Can you work these out from the model? Positions are in its coordinate system, mm. Face numbers are marked on the shaded views. A direction names the side the tool comes from. Give positions to 0.01 mm unless a question says otherwise; leave off trailing zeros. Order: outer loops, then holes, each group sorted by start corner. A loop starts at its lowest first (then second) coordinate and runs counter-clockwise, first axis right, second up. Notation, with made-up numbers: (-30.5, 68) - (18.5, 68) arc R23 ccw to (18.5, 85) - close; hole circle Ø10 at (-36, -0.75). An arc over 180 degrees is marked (long way). Answer as a JSON object with one key per item and string values.
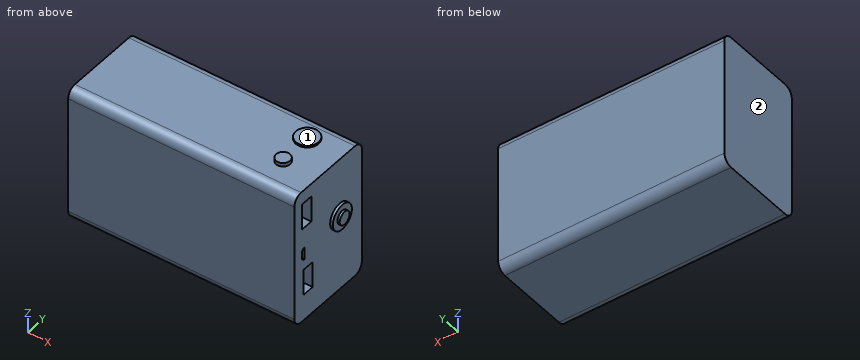
```python
from build123d import *

# Parameters (mm, degrees)
F0_W      = 127
F0_H      = 76.2
F1_DEPTH  = 50.8
F2_R      = 5.08
F3_W      = 7
F3_H      = 14.7
F4_DEPTH  = 16.4084
F5_W      = 7
F5_H      = 14.7
F6_DEPTH  = 16.4084
F8_DEPTH  = 16.4084
F9_R      = 6.390323
F10_DEPTH = 1.016
F11_R     = 7.169195
F12_DEPTH = 1.524
F13_R     = 3.737659
F14_DEPTH = 1.27
F15_R     = 3.927786
F16_DEPTH = 2.032


with BuildPart() as f1:
    # F0 (on Front) → F1 (new body)
    with BuildSketch(Plane.XZ):
        Rectangle(F0_W, F0_H)
    extrude(amount=F1_DEPTH)

    # F2
    f2_edges = [f1.edges().sort_by_distance(p)[0] for p in [
        (0, -50.8, 38.1),
        (0, -50.8, -38.1),
        (0, 0, 38.1),
        (0, 0, -38.1),
    ]]
    fillet(f2_edges, radius=F2_R)

    # F3 (on face) → F4 (cut)
    with BuildSketch(Plane.YZ.offset(63.5)):
        with Locations((-41.585449, 23.312267)):
            Rectangle(F3_W, F3_H)
    extrude(amount=-F4_DEPTH, mode=Mode.SUBTRACT)

    # F5 (on face) → F6 (cut)
    with BuildSketch(Plane.YZ.offset(63.5)):
        with Locations((-40.580612, -15.871216)):
            Rectangle(F5_W, F5_H)
    extrude(amount=-F6_DEPTH, mode=Mode.SUBTRACT)

    # F7 (on face) → F8 (cut)
    with BuildSketch(Plane.YZ.offset(63.5)):
        with BuildLine():
            ThreePointArc((-43.285449, 4.175303), (-44.558241, 3.648095), (-45.085449, 2.375303))
            Line((-45.085449, 2.375303), (-45.085449, -0.874697))
            ThreePointArc((-45.085449, -0.874697), (-44.558241, -2.14749), (-43.285449, -2.674697))
            Line((-43.285449, -2.674697), (-43.285449, 4.175303))
        make_face()
    extrude(amount=-F8_DEPTH, mode=Mode.SUBTRACT)

    # F9 (on face) → F10 (join)
    with BuildSketch(Plane.XY.offset(38.1)):
        with Locations((43.026961, -13.670774)):
            Circle(F9_R)
    extrude(amount=F10_DEPTH)

    # F11 (on face) → F12 (join)
    with BuildSketch(Plane.YZ.offset(63.5)):
        with Locations((-16.692733, 5.036601)):
            Circle(F11_R)
    extrude(amount=F12_DEPTH)

    # F13 (on face) → F14 (join)
    with BuildSketch(Plane.YZ.offset(65.024)):
        with Locations((-16.692733, 5.036601)):
            Circle(F13_R)
    extrude(amount=F14_DEPTH)

    # F15 (on face) → F16 (join)
    with BuildSketch(Plane.XY.offset(38.1)):
        with Locations((43.746475, -32.809857)):
            Circle(F15_R)
    extrude(amount=F16_DEPTH)


solid = f1.part
```
Q1. If we section it at C-C, the plane x = 44: Please give me the cut outline in (y, z).
Recorded:
{"outline": "(-50.8, -33.02) arc R5.08 ccw to (-45.72, -38.1) - (-5.08, -38.1) arc R5.08 ccw to (0, -33.02) - (0, 33.02) arc R5.08 ccw to (-5.08, 38.1) - (-7.35, 38.1) - (-7.35, 39.12) - (-19.99, 39.12) - (-19.99, 38.1) - (-28.89, 38.1) - (-28.89, 40.13) - (-36.73, 40.13) - (-36.73, 38.1) - (-45.72, 38.1) arc R5.08 ccw to (-50.8, 33.02) - close"}
Q2. If we section it at B-B, the plane z = 20: Please give me the cut outline in (x, y).
Recorded:
{"outline": "(-63.5, -50.8) - (63.5, -50.8) - (63.5, -45.09) - (47.09, -45.09) - (47.09, -38.09) - (63.5, -38.09) - (63.5, 0) - (-63.5, 0) - close"}
Q3. I'm going to push flat-ended pins straight in: pin 1 Ø10 at (y, z) = (-26, 6) entering from +X; pin 2 Ø5 at (x, y) = (34, -28) entering from +Z; pin 3 Ø2 at (y, z) = (-44.5, -0.5) entering from +X. Where does each tip first touch, or does it pass through?
Recorded:
{"pin 1": "stops at x = 65.02", "pin 2": "stops at z = 38.1", "pin 3": "stops at x = 63.5"}
Q4. If we section it at A-A, the plane x = -5: Please give me the cut outline in (y, z), then the cut area to 3 significant figures.
Recorded:
{"outline": "(-50.8, -33.02) arc R5.08 ccw to (-45.72, -38.1) - (-5.08, -38.1) arc R5.08 ccw to (0, -33.02) - (0, 33.02) arc R5.08 ccw to (-5.08, 38.1) - (-45.72, 38.1) arc R5.08 ccw to (-50.8, 33.02) - close", "area": "3,850 mm^2"}
Q5. I need wall thicknesses on L1, parallel to Z at x = -2.5, y = -24.5; L2, parallel to X at y = -17.5, z = -31; L3, parallel to Z at x = 45, y = -19. Which ranges of each line are inside material? Lowest first, please.
Recorded:
{"L1": "z = -38.1 to 38.1", "L2": "x = -63.5 to 63.5", "L3": "z = -38.1 to 39.12"}
Q6. Which directions (+Z, -Z, +X, -X, +Y, -Y) give clear straight access to the entire face, cutting with the end or side of a thin tool? Please do the marked faces 1 and 2.
Recorded:
{"face 1": "+Z, +X, -X, +Y", "face 2": "+Z, -Z, -X, +Y, -Y"}
